from build123d import *

# Parameters (mm, degrees)
SKETCH1_W           = 4
SKETCH1_H           = 17
BOSS_EXTRUDE1_DEPTH = 6
SKETCH2_W           = 2.8
SKETCH2_H           = 6.5
SKETCH2_W_2         = 1.5
SKETCH2_H_2         = 2.75
CUT_EXTRUDE1_DEPTH  = 19.466185313
CUT_EXTRUDE2_DEPTH  = 19.466185313
SKETCH4_W           = 2
SKETCH4_H           = 2.75
BOSS_EXTRUDE2_DEPTH = 2
SKETCH6_W           = 1.5
SKETCH6_H           = 1.5
SKETCH6_H_2         = 0.75
CUT_EXTRUDE3_DEPTH  = 2
SKETCH7_W           = 1.3
SKETCH7_H           = 6.5
BOSS_EXTRUDE3_DEPTH = 2.8
SKETCH8_R           = 1.5
CUT_EXTRUDE4_DEPTH  = 10


with BuildPart() as part:
    # Sketch1 → Boss-Extrude1 (new body)
    with BuildSketch(Plane.XY):
        with Locations((2, 8.5)):
            Rectangle(SKETCH1_W, SKETCH1_H)
    extrude(amount=BOSS_EXTRUDE1_DEPTH)

    # Sketch2 → Cut-Extrude1 (cut, through all)
    with BuildSketch(Plane.XY.offset(6)):
        with Locations((2.6, 9.25)):
            Rectangle(SKETCH2_W, SKETCH2_H)
        with Locations((3.25, 3.875)):
            Rectangle(SKETCH2_W_2, SKETCH2_H_2)
    extrude(amount=-CUT_EXTRUDE1_DEPTH, mode=Mode.SUBTRACT)

    # Sketch3 → Cut-Extrude2 (cut, through all)
    with BuildSketch(Plane.ZY):
        Polygon((0, 15.25), (0.75, 14.25), (0.75, 15.25), (2, 15.25), (2, 1.75), (0.75, 1.75), (0.75, 2.75), (0, 1.75), align=None)
    extrude(amount=-CUT_EXTRUDE2_DEPTH, mode=Mode.SUBTRACT)

    # Sketch4 → Boss-Extrude2 (add)
    with BuildSketch(Plane(origin=(4, 0, 0), x_dir=(0, 0, -1), z_dir=(1, 0, 0))):
        with Locations((-5, 3.875)):
            Rectangle(SKETCH4_W, SKETCH4_H)
    extrude(amount=-BOSS_EXTRUDE2_DEPTH)

    # Sketch6 → Cut-Extrude3 (cut)
    with BuildSketch(Plane(origin=(0, 0, 2), x_dir=(-1, 0, 0), z_dir=(0, 0, -1))):
        with Locations((-3.25, 13.25)):
            Rectangle(SKETCH6_W, SKETCH6_H)
        with Locations((-3.25, 5.625)):
            Rectangle(SKETCH6_W, SKETCH6_H_2)
    extrude(amount=-CUT_EXTRUDE3_DEPTH, mode=Mode.SUBTRACT)

    # Sketch7 → Boss-Extrude3 (add)
    with BuildSketch(Plane(origin=(1.2, 0, 0), x_dir=(0, 0, -1), z_dir=(1, 0, 0))):
        with Locations((-5.35, 9.25)):
            Rectangle(SKETCH7_W, SKETCH7_H)
    extrude(amount=BOSS_EXTRUDE3_DEPTH)

    # Sketch8 → Cut-Extrude4 (cut)
    with BuildSketch(Plane(origin=(0, 0, 4.7), x_dir=(-1, 0, 0), z_dir=(0, 0, -1))):
        with Locations((-2.7, 9)):
            Circle(SKETCH8_R)
    extrude(amount=-CUT_EXTRUDE4_DEPTH, mode=Mode.SUBTRACT)


solid = part.part
Geometry check sheet. Reference: the model listing, model coordinates, mm. A direction names the side the tool comes from. Give positions to 0.01 mm unless a question says otherwise; leave off trailing zeros. Loops run counter-clockwise (first coordinate to the right, second up) from the corner with the lowest first, then second, coordinate; pieces in that order, holes last. Notation, with made-up numbers: M 5.25,-0.5 L 11.25,-0.5 A21 cw 11.25,10.5 Z; hole C 9.25,-1 d1. An arc over 180 degrees is marked long. Write each question's results on one line, items separated by ' | '.
1) Section check B-B, the plane x = 1.5. Record the boundary of the cut face in (y, z).
Answers follow:
outline: M 0,0 L 1.75,0 L 2.75,0.75 L 1.75,0.75 L 1.75,2 L 6,2 L 6,4.7 L 8.1,4.7 L 8.1,6 L 0,6 Z; M 9.9,4.7 L 12.5,4.7 L 12.5,2 L 15.25,2 L 15.25,0.75 L 14.25,0.75 L 15.25,0 L 17,0 L 17,6 L 9.9,6 Z
2) Gauge pin test, flat ends, axial feed: pin 1 (1.3 mm diameter, centred on y = 10, z = 2.5, fed in from +X); pin 2 (1.4 mm diameter, centred on x = 2.5, y = 7.5, fed in from -Z); pin 3 (1.2 mm diameter, centred on x = 3, y = 4, fed in from -Z). Record the tip position at first contact, or that the pin passes through.
Answers follow:
pin 1: x = 1.2 | pin 2: z = 4.7 | pin 3: z = 2
3) Section check C-C, the plane y = 4. Record the boundary of the cut face in (x, z).
Answers follow:
outline: M 0,2 L 2.5,2 L 2.5,4 L 4,4 L 4,6 L 0,6 Z
4) Release check for a two-part mould opening along Y. For faces 5 (the face through (3, 13, 4)), 6 (the face through (4, 3.3, 4.4)), 7 (the face through (2.5, 13, 3)), 8 (the face through (2, 0, 3)) record: +Y half, -Y half, draft (parallel to the pull), parting line (faces both ways), or undercut.
Answers follow:
face 5: undercut | face 6: draft | face 7: undercut | face 8: -Y half
5) Tool access check on faces 1 (the face through (2, 15, 0.75)), 2 (the face through (3, 2.5, 3)), 3 (the face through (2, 1, 0)), 4 (the face through (1.972, 14.757, 0.37)). Record the directions out of +Z, -Z, +X, -X, +Y, -Y that give a thin tool (end or side, any length) a straight path to the whole face; none if there is none.
Answers follow:
face 1: +X, -X | face 2: -Z, +X | face 3: -Z, +X, -X, +Y, -Y | face 4: -Z, +X, -X
6) Thickness scan on line 1 (Y direction, x = 3.4, z = 4.25); line 2 (Y direction, x = 2.7, z = 5.5); line 3 (X direction, y = 3.5, z = 2.35). Record the ranges inside material, lowest first.
Answers follow:
line 1: 0 to 6, 12.5 to 17 | line 2: 0 to 7.5, 10.5 to 17 | line 3: 0 to 2.5
7) Section check D-D, the plane x = 0.7. Record the boundary of the cut face in (y, z), plus the area to 4 significant figures.
Answers follow:
outline: M 0,0 L 1.75,0 L 2.75,0.75 L 1.75,0.75 L 1.75,2 L 15.25,2 L 15.25,0.75 L 14.25,0.75 L 15.25,0 L 17,0 L 17,6 L 0,6 Z | area: 75.75 mm2
8) Section check A-A, the plane z = 1.6. Record the boundary of the cut face in (x, y), plus the area to 3 significant figures.
Answers follow:
outline: M 0,0 L 4,0 L 4,1.75 L 0,1.75 Z; M 0,15.25 L 4,15.25 L 4,17 L 0,17 Z | area: 14.0 mm2
